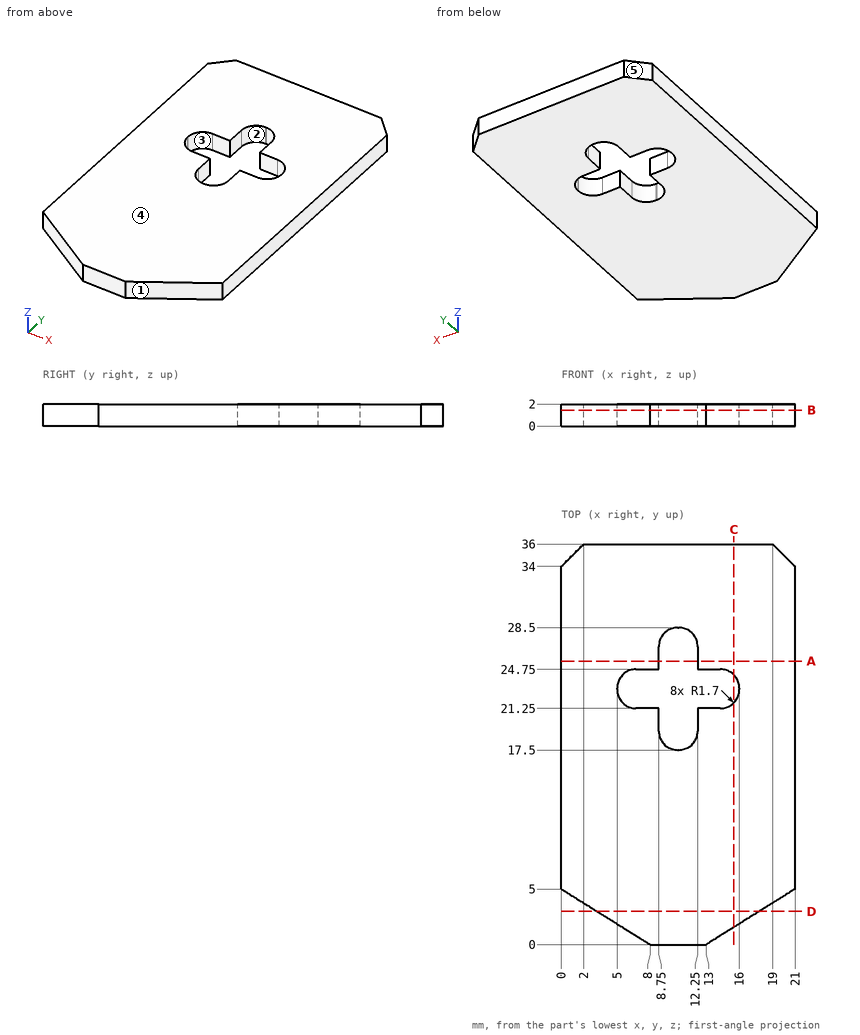
Source: three-view drawing plus pictorial views. Frame: mm from the lowest corner of the part. A direction names the side the tool comes from. Give positions to 0.01 mm unless a question says otherwise; leave off trailing zeros. Order: outer loops, then holes, each group sorted by start corner. A loop starts at its lowest first (then second) coordinate and runs counter-clockwise, first axis right, second up. Notation, with made-up numbers: (28, -36.5) - (84, -36.5) arc R24 cw to (84, -14.5) - close; hole circle Ø2 at (-22.75, -2). An arc over 180 degrees is marked (long way). Answer as a JSON object with one key per item and string values. Group by question number.
Q1. Set-up query: the marked faces 1 and 2. Return all of +Z, -Z, +X, -X, +Y, -Y with unobstructed straight access to the full face (end or side cutting, diameter ignored); none if empty.
Q2. Mould query, pull axis X, two halves, no side actions, for the marked faces 3, 4 and 5. Classes: pulls with the +X half, pulls with the -X half, needs draft (parallel to the pull), parting line crosses it, or undercut.
Q3. Cut plane C-C, the plane x = 15.5. Output: boundary loops of the cut face in (y, z).
Q4. Cut plane D-D, the plane y = 3. Output: boundary loops of the cut face in (x, z), then the cut area to 3 significant figures.
Q5. Line query: probe 1 along Y at (x, z) = (8, 1.3); probe 2 along X at (y, z) = (19.5, 0.15); probe 3 along X at (y, z) = (24.5, 1.85). Output: solid intervals per line, ascending.
Q6. First-contact query: pin 1 Ø1 at (x, z) = (5, 0.5) entering from -Y. Flat tip, straight axial feed; report the tip coordinate or a pass-through.
Q7. Cut plane A-A, the plane y = 25.5. Output: boundary loops of the cut face in (x, z).
Q8. Cut plane B-B, the plane z = 1.45. Output: boundary loops of the cut face in (x, y), then the cut area to 3 significant figures.
Results:
{
 "1": {"face 1": "+Z, -Z, +X, -Y", "face 2": "+Z, -Z"},
 "2": {"face 3": "undercut", "face 4": "needs draft", "face 5": "pulls with the -X half"},
 "3": {"outline": "(1.56, 0) - (21.75, 0) - (21.75, 2) - (1.56, 2) - close; (24.25, 0) - (36, 0) - (36, 2) - (24.25, 2) - close"},
 "4": {"outline": "(3.2, 0) - (17.8, 0) - (17.8, 2) - (3.2, 2) - close", "area": "29.2 mm^2"},
 "5": {"probe 1": "0 to 21.25, 24.75 to 36", "probe 2": "0 to 8.75, 12.25 to 21", "probe 3": "0 to 5.81, 15.19 to 21"},
 "6": {"pin 1": "y = 1.56"},
 "7": {"outline": "(0, 0) - (8.75, 0) - (8.75, 2) - (0, 2) - close; (12.25, 0) - (21, 0) - (21, 2) - (12.25, 2) - close"},
 "8": {"outline": "(0, 5) - (8, 0) - (13, 0) - (21, 5) - (21, 34) - (19, 36) - (2, 36) - (0, 34) - close; hole (5, 22.95) arc R1.7 ccw to (6.7, 21.25) - (8.75, 21.25) - (8.75, 19.2) arc R1.7 ccw to (10.45, 17.5) - (10.55, 17.5) arc R1.7 ccw to (12.25, 19.2) - (12.25, 21.25) - (14.3, 21.25) arc R1.7 ccw to (16, 22.95) - (16, 23.05) arc R1.7 ccw to (14.3, 24.75) - (12.25, 24.75) - (12.25, 26.8) arc R1.7 ccw to (10.55, 28.5) - (10.45, 28.5) arc R1.7 ccw to (8.75, 26.8) - (8.75, 24.75) - (6.7, 24.75) arc R1.7 ccw to (5, 23.05) - close", "area": "652 mm^2"}
}
